from build123d import *

# Parameters (mm, degrees)
F0_W     = 508
F0_H     = 50.8
F1_DEPTH = 3.175
F2_W     = 101.6
F2_H     = 3.175
F3_DEPTH = 25.4
F4_W     = 101.6
F4_H     = 3.175
F5_DEPTH = 25.4
F6_W     = 127
F6_H     = 3.175
F7_DEPTH = 25.4


with BuildPart() as f1:
    # F0 (on Top) → F1 (new body)
    with BuildSketch(Plane.XY):
        with Locations((254, 25.4)):
            Rectangle(F0_W, F0_H)
    extrude(amount=F1_DEPTH)

    # F2 (on face) → F3 (cut)
    with BuildSketch(Plane.XY.offset(3.175)):
        with Locations((152.4, 1.5875)):
            Rectangle(F2_W, F2_H)
        with Locations((355.6, 1.5875)):
            Rectangle(F2_W, F2_H)
    extrude(amount=-F3_DEPTH, mode=Mode.SUBTRACT)

    # F4 (on face) → F5 (cut)
    with BuildSketch(Plane.XY.offset(3.175)):
        with Locations((152.4, 49.2125)):
            Rectangle(F4_W, F4_H)
        with Locations((355.6, 49.2125)):
            Rectangle(F4_W, F4_H)
    extrude(amount=-F5_DEPTH, mode=Mode.SUBTRACT)

    # F6 (on face) → F7 (cut)
    with BuildSketch(Plane.XY.offset(3.175)):
        with Locations((444.5, 25.4)):
            Rectangle(F6_W, F6_H)
    extrude(amount=-F7_DEPTH, mode=Mode.SUBTRACT)


solid = f1.part
Check sheet for the modelled part. Datum: model origin and axes. Units: mm. Coordinates: 2 decimals unless noted, no trailing zeros. Write each loop counter-clockwise with the first axis right and the second up, starting at its lowest first coordinate (ties: lowest second). Pieces come first, ordered by that corner, then holes.
Item 1: Scan lines: probe 1 along X at (y, z) = (3, 0.5); probe 2 along Y at (x, z) = (423.5, 0.3); probe 3 along Y at (x, z) = (141.5, 1) (3 decimals). Record each from-to range of solid material in increasing order.
Numbers:
probe 1: x = 0 to 101.6, 203.2 to 304.8, 406.4 to 508
probe 2: y = 0 to 23.81, 26.99 to 50.8
probe 3: y = 3.175 to 47.625
Item 2: Cross-section at A-A on x = 447. Record the boundary of the cut face in (y, z) (1 decimal).
Numbers:
outline: (0, 0) - (23.8, 0) - (23.8, 3.2) - (0, 3.2) - close; (27, 0) - (50.8, 0) - (50.8, 3.2) - (27, 3.2) - close
Item 3: Depth check by flat-ended pin: pin 1 Ø3 at (x, y) = (367, 35.5) entering from -Z; pin 2 Ø1.6 at (x, z) = (378.5, 2) entering from +Y (3 decimals); pin 3 Ø1 at (x, z) = (139.5, 1.5) entering from -Y (3 decimals). Enter the tip coordinate at first touch or a pass-through.
Numbers:
pin 1: stops at z = 0
pin 2: stops at y = 47.625
pin 3: stops at y = 3.175
Item 4: Cross-section at C-C on x = 124. Record the boundary of the cut face in (y, z) (3 decimals), then the cut area to 3 significant figures.
Numbers:
outline: (3.175, 0) - (47.625, 0) - (47.625, 3.175) - (3.175, 3.175) - close
area: 141 mm2
Item 5: Cross-section at B-B on z = 1.85. Record the boundary of the cut face in (x, y) (1 decimal), then the cut area to 3 significant figures.
Numbers:
outline: (0, 0) - (101.6, 0) - (101.6, 3.2) - (203.2, 3.2) - (203.2, 0) - (304.8, 0) - (304.8, 3.2) - (406.4, 3.2) - (406.4, 0) - (508, 0) - (508, 23.8) - (381, 23.8) - (381, 27) - (508, 27) - (508, 50.8) - (406.4, 50.8) - (406.4, 47.6) - (304.8, 47.6) - (304.8, 50.8) - (203.2, 50.8) - (203.2, 47.6) - (101.6, 47.6) - (101.6, 50.8) - (0, 50.8) - close
area: 24,100 mm2
